```python
from build123d import *
from build123d.topology import SkipClean

# Parameters (mm, degrees)
BOSS_EXTRUDE1_DEPTH = 1.27
BOSS_EXTRUDE2_START = 5.08
BOSS_EXTRUDE2_DEPTH = 5.08
SKETCH3_R           = 9.525
BOSS_EXTRUDE3_DEPTH = 5.08
CUT_EXTRUDE2_START  = -4.85
SKETCH7_R           = 2.85
CUT_EXTRUDE2_DEPTH  = 4.85


with BuildPart() as part:
    # Sketch1 → Boss-Extrude1 (new body)
    with BuildSketch(Plane.XZ.offset(-243.34664948)):
        with BuildLine():
            ThreePointArc((170.976440709, 548.746338149), (161.451440709, 536.449616024), (170.976440709, 524.1528939))
            ThreePointArc((170.976440709, 524.1528939), (174.151440709, 523.749616024), (177.326440709, 524.1528939))
            ThreePointArc((177.326440709, 524.1528939), (186.851440709, 536.449616024), (177.326440709, 548.746338149))
            ThreePointArc((177.326440709, 548.746338149), (174.151440709, 549.149616024), (170.976440709, 548.746338149))
        make_face()
    extrude(amount=BOSS_EXTRUDE1_DEPTH)

    # Sketch2 → Boss-Extrude2 (add)
    with SkipClean():  # the faces are left unmerged after this step: merging them gives an invalid solid
        with BuildSketch(Plane(origin=(0, 243.34664948, 0), x_dir=(1, 0, 0), z_dir=(0, 1, 0)).offset(BOSS_EXTRUDE2_START)):
            with BuildLine():
                Line((177.326440709, -524.1528939), (177.326440709, -548.746338149))
                ThreePointArc((177.326440709, -548.746338149), (186.851440709, -536.449616024), (177.326440709, -524.1528939))
            make_face()
            with BuildLine():
                Line((170.976440709, -548.746338149), (170.976440709, -524.1528939))
                ThreePointArc((170.976440709, -524.1528939), (161.451440709, -536.449616024), (170.976440709, -548.746338149))
            make_face()
        extrude(amount=-BOSS_EXTRUDE2_DEPTH)

    # Sketch3 → Boss-Extrude3 (add)
    with SkipClean():  # the faces are left unmerged after this step: merging them gives an invalid solid
        with BuildSketch(Plane.XZ.offset(-242.07664948)):
            with Locations(Location((174.151440709, 536.449616024, 0), (0, 0, 270))):
                Circle(SKETCH3_R)
        extrude(amount=BOSS_EXTRUDE3_DEPTH)

    # Sketch7 → Cut-Extrude2 (cut)
    with SkipClean():  # the faces are left unmerged after this step: merging them gives an invalid solid
        with BuildSketch(Plane.XZ.offset(-236.99664948).offset(CUT_EXTRUDE2_START)):
            with Locations(Location((174.151440709, 536.449616024, 0), (0, 0, 270))):
                Circle(SKETCH7_R)
        extrude(amount=CUT_EXTRUDE2_DEPTH, mode=Mode.SUBTRACT)


solid = part.part
```
Can you work these out from the model? Positions are in its coordinate system, mm. A direction names the side the tool comes from. Give positions to 0.01 mm unless a question says otherwise; leave off trailing zeros. Order: outer loops, then holes, each group sorted by start corner. A loop starts at its lowest first (then second) coordinate and runs counter-clockwise, first axis right, second up. Notation, with made-up numbers: M 19.5,54.25 L 74.5,54.25 A14 cw 74.5,63.25 Z; hole C -29,17 d6. An arc over 180 degrees is marked long. Write item = value, one per line. Start each with the question number.
Q1. I need wall thicknesses on probe 1 along Y at (x, z) = (166.75, 529.75); probe 2 along X at (y, z) = (247, 526.5); probe 3 along Y at (x, z) = (174, 536.5). Which ranges of each line are inside material? Lowest first, please. Write a range as [from, to].
Q2. Will these pins go through, and if not, where does the flat tip stop? pin 1 Ø1.7 at (x, z) = (175, 536) entering from -Y; pin 2 Ø3 at (y, z) = (238.5, 532.5) entering from -X; pin 3 Ø6 at (y, z) = (243, 541.5) entering from +X.
Q3. Suppose I cut it at A-A (x = 182.25). Write out the boundary of the cut face in (y, z), plus the area to 3 significant figures.
Q4. Suppose I cut it at C-C (y = 247). Write out the boundary of the cut face in (x, z).
Q5. We'd pull the mould along Z, two halves only. Please class faces 4 (the cylindrical face through (177.012, 239.572, 527.364)), 5 (the flat face through (177.326, 246, 536)), 6 (the flat face through (174, 241.847, 536)): pulls with the +Z half, pulls with the -Z half, needs draft (parallel to the pull), parting line crosses it, or undercut.
Q6. Suppose I cut it at B-B (z = 534). Write out the boundary of the cut face in (x, y).
Q7. For faces 1 (the flat face through (181, 248.427, 536)), 2 (the cylindrical face through (175.01, 239.46, 533.73)), 3 (the flat face through (174, 243.347, 537)), which set-ups out of +Z, -Z, +X, -X, +Y, -Y let a thin tool reach every point of the face, with its end or its side?
Q8. Suppose I cut it at D-D (y = 242.5). Write out the boundary of the cut face in (x, z).
Check result:
q1.probe_1 = [242.08, 248.43]
q1.probe_2 = [166.26, 170.98], [177.33, 182.04]
q1.probe_3 = [241.85, 243.35]
q2.pin_1 = 241.85
q2.pin_2 = 164.95
q2.pin_3 = 186.68
q3.outline = M 237,531.44 L 242.08,531.44 L 242.08,526.67 L 248.43,526.67 L 248.43,546.23 L 242.08,546.23 L 242.08,541.46 L 237,541.46 Z
q3.area = 175 mm2
q4.outline = M 170.98,524.15 L 170.98,548.75 A12.7 ccw Z; M 177.33,524.15 A12.7 ccw 177.33,548.75 Z
q5.face_4 = parting line crosses it
q5.face_5 = needs draft
q5.face_6 = undercut
q6.outline = M 161.69,242.08 L 164.95,242.08 L 164.95,237 L 172.69,237 L 172.69,241.85 L 175.61,241.85 L 175.61,237 L 183.36,237 L 183.36,242.08 L 186.61,242.08 L 186.61,248.43 L 177.33,248.43 L 177.33,243.35 L 170.98,243.35 L 170.98,248.43 L 161.69,248.43 Z
q7.face_1 = +Z, -Z, +X, -X, +Y
q7.face_2 = -Y
q7.face_3 = +Z, -Z, +Y
q8.outline = C 174.15,536.45 d25.4
